Part model, mm, in its own coordinate system. A direction names the side the tool comes from. Round coordinates to 2 decimals unless told otherwise and drop trailing zeros. Write each loop counter-clockwise with the first axis right and the second up, starting at its lowest first coordinate (ties: lowest second). Pieces come first, ordered by that corner, then holes. Notation, with made-up numbers: M 34,31 L 73,31 A11 ccw 73,49 Z; hole C 79,79 d1. An arc over 180 degrees is marked long. Use one line per item in the form item = value. Start each with the question number.
Item 1: Probe L1, parallel to Z at x = -6.5, y = 17.5; L2, parallel to X at y = 1, z = 12; L3, parallel to Z at x = 0.5, y = 14.25. List the from-to ranges inside material, lowest first.
Item 2: Mould opens along Z. For faces 6 (the face through (0, 14, 25)), 7 (the face through (25, 14, 0)), 8 (the face through (0, 5, 26)) say: +Z half, -Z half, draft (parallel to the pull), parting line (faces both ways), or undercut.
Item 3: Cut at D-D, the plane x = -15. Give the cut face in (y, z).
Item 4: Flat gauge pins, fed straight in: pin 1 Ø2 at (x, z) = (1.5, 18.5) entering from -Y; pin 2 Ø24 at (x, z) = (-9, -5.5) entering from +Y; pin 3 Ø1.9 at (x, z) = (-12, 12) entering from -Y (3 decimals). Where does each tip first touch, or does it go through?
Item 5: Cut at C-C, the plane y = 8.5. Give the cut face in (x, z).
Item 6: Cut at A-A, the plane x = 0. Give the cut face in (y, z).
Item 7: Which spindle directions (+Z, -Z, +X, -X, +Y, -Y) get a long thin tool onto all of the face, cutting with end or side? Do faces 1 (the face through (-25, 10, 22.5)), 2 (the face through (-0.3, 5.8, -24)), 3 (the face through (-22.5, 10, -25)), 4 (the face through (0, 5, -26)), 5 (the face through (-11.93, 0.99, -13.6)). Say none if no direction does.
Item 8: Cut at B-B, the plane z = 19. Give the cut face in (x, y), then the cut area to 3 significant figures.
from build123d import *

# Parameters (mm, degrees)
SKETCH_1_W               = 52
SKETCH_1_H               = 52
SKETCH_1_R               = 1.6
SKETCH_1_W_2             = 20
SKETCH_1_H_2             = 20
EXTRUDE_5_DEPTH          = 20
SHELL_6_T                = -2
SKETCH_4_W               = 50
SKETCH_4_H               = 50
SKETCH_4_W_2             = 48
SKETCH_4_H_2             = 48
CUT_EXTRUDE_4_DEPTH      = 4
CUT_EXTRUDE_5_DEPTH      = 60.799665551
CUT_EXTRUDE_5_DEPTH_BACK = 60.799665551
SKETCH_5_W               = 45
SKETCH_5_H               = 8
CUT_EXTRUDE_6_DEPTH      = 60.799665551
CUT_EXTRUDE_6_DEPTH_BACK = 60.799665551
SKETCH_6_W               = 45
SKETCH_6_H               = 8
SKETCH_7_R               = 14.142135624
CUT_EXTRUDE_7_DEPTH      = 10


with BuildPart() as part:
    # 草图1 → 凸台-拉伸5 (new body)
    with BuildSketch(Plane(origin=(0, 0, 0), x_dir=(1, 0, 0), z_dir=(0, 1, 0))):
        Rectangle(SKETCH_1_W, SKETCH_1_H)
        with Locations(Location((-12, 12, 0), (0, 0, 270))):
            Circle(SKETCH_1_R, mode=Mode.SUBTRACT)
        with Locations(Location((12, 12, 0), (0, 0, 270))):
            Circle(SKETCH_1_R, mode=Mode.SUBTRACT)
        with Locations(Location((12, -12, 0), (0, 0, 270))):
            Circle(SKETCH_1_R, mode=Mode.SUBTRACT)
        with Locations(Location((-12, -12, 0), (0, 0, 270))):
            Circle(SKETCH_1_R, mode=Mode.SUBTRACT)
        Rectangle(SKETCH_1_W_2, SKETCH_1_H_2, mode=Mode.SUBTRACT)
    extrude(amount=EXTRUDE_5_DEPTH)

    # 抽壳6
    shell_6_openings = [part.faces().sort_by_distance(p)[0] for p in [
        (-12, 10, 10.4),
        (-10, 10, 0),
        (0, 10, 10),
        (10, 10, 0),
        (0, 10, -10),
        (12, 10, -13.6),
        (-12, 10, -13.6),
        (0, 20, -25.264608948),
        (12, 10, 10.4),
    ]]
    offset(amount=SHELL_6_T, openings=shell_6_openings, kind=Kind.INTERSECTION)

    # 草图4 → 切除-拉伸4 (cut)
    with BuildSketch(Plane(origin=(0, 20, 0), x_dir=(1, 0, 0), z_dir=(0, 1, 0))):
        Rectangle(SKETCH_4_W, SKETCH_4_H)
        Rectangle(SKETCH_4_W_2, SKETCH_4_H_2, mode=Mode.SUBTRACT)
    extrude(amount=-CUT_EXTRUDE_4_DEPTH, mode=Mode.SUBTRACT)

    # 草图5 → 切除-拉伸5 (cut, two sides: drawn at the far end of the back side and taken through both)
    with BuildSketch(Plane.XY.offset(-24).offset(-CUT_EXTRUDE_5_DEPTH_BACK)):
        with Locations((0, 10)):
            Rectangle(SKETCH_5_W, SKETCH_5_H)
    extrude(amount=CUT_EXTRUDE_5_DEPTH + CUT_EXTRUDE_5_DEPTH_BACK, mode=Mode.SUBTRACT)

    # 草图6 → 切除-拉伸6 (cut, two sides: drawn at the far end of the back side and taken through both)
    with BuildSketch(Plane(origin=(-24, 0, 0), x_dir=(0, 0, -1), z_dir=(1, 0, 0)).offset(-CUT_EXTRUDE_6_DEPTH_BACK)):
        with Locations((0, 10)):
            Rectangle(SKETCH_6_W, SKETCH_6_H)
    extrude(amount=CUT_EXTRUDE_6_DEPTH + CUT_EXTRUDE_6_DEPTH_BACK, mode=Mode.SUBTRACT)

    # 草图7 → 切除-拉伸7 (cut)
    with BuildSketch(Plane.XZ):
        with Locations(Location((0, 0, 0), (0, 0, 270))):
            Circle(SKETCH_7_R)
    extrude(amount=-CUT_EXTRUDE_7_DEPTH, mode=Mode.SUBTRACT)


solid = part.part
Model answer:
q1.L1 = -26 to -25, 25 to 26
q1.L2 = -26 to -13.6, -10.4 to -7.48, 7.48 to 10.4, 13.6 to 26
q1.L3 = -26 to -24, 24 to 26
q2.face_6 = draft
q2.face_7 = undercut
q2.face_8 = +Z half
q3.outline = M 0,-26 L 6,-26 L 6,-24 L 2,-24 L 2,24 L 6,24 L 6,26 L 0,26 Z; M 14,-26 L 20,-26 L 20,-25 L 16,-25 L 16,-24 L 14,-24 Z; M 14,24 L 16,24 L 16,25 L 20,25 L 20,26 L 14,26 Z
q4.pin_1 = 0
q4.pin_2 = 2
q4.pin_3 = through
q5.outline = M -26,-26 L -22.5,-26 L -22.5,-24 L -24,-24 L -24,-22.5 L -26,-22.5 Z; M -26,22.5 L -24,22.5 L -24,24 L -22.5,24 L -22.5,26 L -26,26 Z; M 22.5,-26 L 26,-26 L 26,-22.5 L 24,-22.5 L 24,-24 L 22.5,-24 Z; M 22.5,24 L 24,24 L 24,22.5 L 26,22.5 L 26,26 L 22.5,26 Z
q6.outline = M 0,-26 L 6,-26 L 6,-24 L 2,-24 L 2,-14.14 L 0,-14.14 Z; M 0,14.14 L 2,14.14 L 2,24 L 6,24 L 6,26 L 0,26 Z; M 14,-26 L 20,-26 L 20,-25 L 16,-25 L 16,-24 L 14,-24 Z; M 14,24 L 16,24 L 16,25 L 20,25 L 20,26 L 14,26 Z
q7.face_1 = +X, -X
q7.face_2 = +Y
q7.face_3 = +Z, -Z
q7.face_4 = -Z, +X, -X, +Y, -Y
q7.face_5 = +Y, -Y
q8.outline = M -26,0 L 26,0 L 26,6 L 24,6 L 24,2 L -24,2 L -24,6 L -26,6 Z; M -26,14 L -24,14 L -24,16 L -25,16 L -25,20 L -26,20 Z; M 24,14 L 26,14 L 26,20 L 25,20 L 25,16 L 24,16 Z
q8.area = 136 mm²
